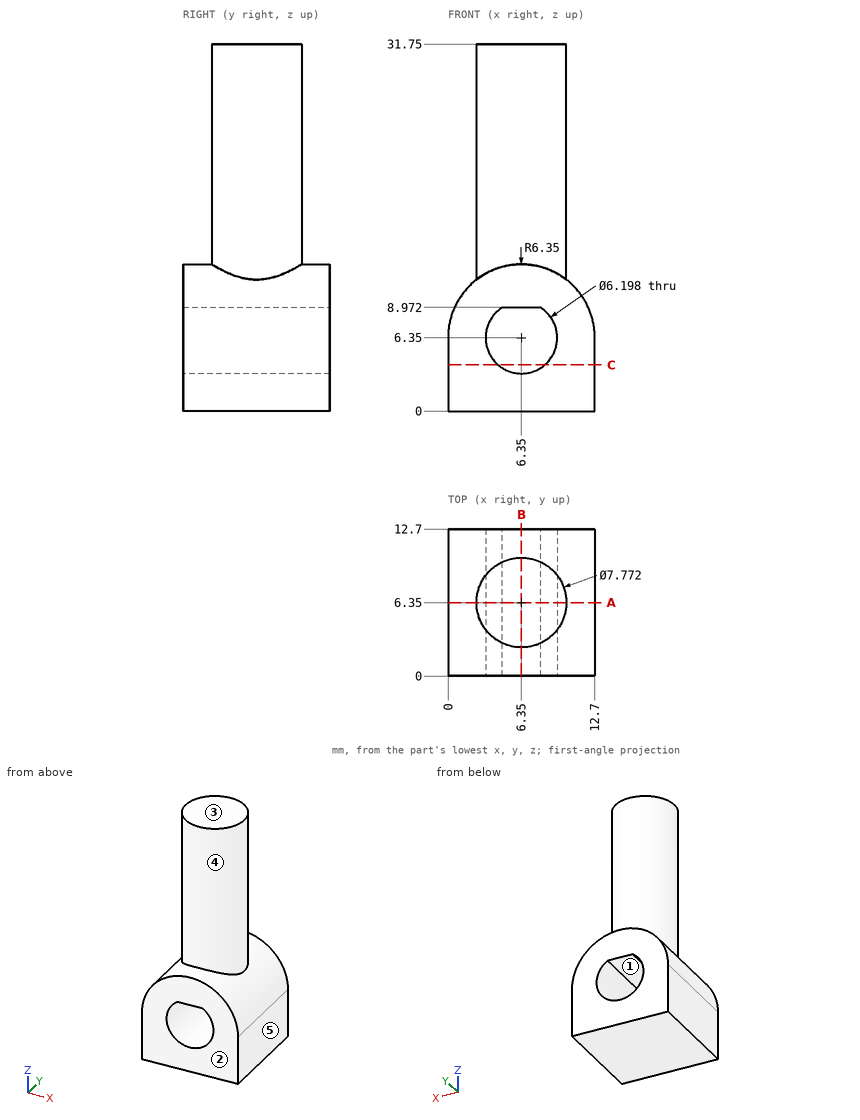
For this review, use the dimensioned drawing (mm, ordinates from the lowest corner) and the shaded views. A direction names the side the tool comes from. Round coordinates to 2 decimals unless told otherwise and drop trailing zeros. Write each loop counter-clockwise with the first axis right and the second up, starting at its lowest first coordinate (ties: lowest second). Pieces come first, ordered by that corner, then holes. Notation, with made-up numbers: (-7, 37.25) -> (48, 37.25) arc R12 cw to (48, 60.25) -> close; hole circle Ø11 at (42, 9). An arc over 180 degrees is marked (long way). Use CSV: the item, a comma, the result in double quotes.
(1) Consider section B-B, the plane x = 6.35. Give the boundary of the cut face in (y, z).
Computed values:
outline,"(0, 0) -> (12.7, 0) -> (12.7, 3.25) -> (0, 3.25) -> close; (0, 8.97) -> (12.7, 8.97) -> (12.7, 12.7) -> (10.24, 12.7) -> (10.24, 31.75) -> (2.46, 31.75) -> (2.46, 12.7) -> (0, 12.7) -> close"
(2) For the marked faces 4 and 5, list the 3-axis set-ups (+Z, -Z, +X, -X, +Y, -Y) from which the entire face can be reached by the end or side of a thin tool; tool diameter is ignored.
Computed values:
face 4,"+Z"
face 5,"+Z, -Z, +X, +Y, -Y"
(3) To check wall thickness, follow L1, parallel to X at y = 4, z = 17.5 (1 decimal); L2, parallel to Z at x = 5.5, y = 0.75; L3, parallel to Z at x = 5.75, y = 0.75. State the ranges of each line that lie inside material, in increasing order. Write a range as [from, to].
Computed values:
L1,"[3.3, 9.4]"
L2,"[0, 3.37], [8.97, 12.64]"
L3,"[0, 3.31], [8.97, 12.67]"
(4) Draft analysis for pull direction Z (two halves, no side actions). For the marked faces 1, 2 and 3, state which applies: +Z half, -Z half, draft (parallel to the pull), parting line (faces both ways), or undercut.
Computed values:
face 1,"undercut"
face 2,"draft"
face 3,"+Z half"
(5) Consider section A-A, the plane y = 6.35. Give the boundary of the cut face in (x, z), plus the area to 3 significant figures.
Computed values:
outline,"(0, 0) -> (12.7, 0) -> (12.7, 6.35) arc R6.35 ccw to (10.24, 11.37) -> (10.24, 31.75) -> (2.46, 31.75) -> (2.46, 11.37) arc R6.35 ccw to (0, 6.35) -> close; hole (4.7, 8.97) arc R3.1 ccw (long way) to (8, 8.97) -> close"
area,"266 mm²"
(6) Consider section C-C, the plane z = 4. Give the boundary of the cut face in (x, y), plus the area to 3 significant figures.
Computed values:
outline,"(0, 0) -> (4.33, 0) -> (4.33, 12.7) -> (0, 12.7) -> close; (8.37, 0) -> (12.7, 0) -> (12.7, 12.7) -> (8.37, 12.7) -> close"
area,"110 mm²"
(7) Clearance check with flat-ended pins moving along their axes: P1, Ø1, axis at x = 10, y = 10, coming from the +Z side; P2, Ø4, axis at y = 10, z = 24.5, coming from the -X side; P3, Ø3.5, axis at x = 6.35, z = 6.35, coming from the +Y side. State where each tip first meets the part, or that it passes through.
Computed values:
P1,"z = 11.86"
P2,"x = 2.83"
P3,"through"
